Check sheet for the drawn part. Datum: minimum x, y, z corner. Units: mm. Round coordinates to 2 decimals unless told otherwise and drop trailing zeros. Write each loop counter-clockwise with the first axis right and the second up, starting at its lowest first coordinate (ties: lowest second). Pieces come first, ordered by that corner, then holes. Notation, with made-up numbers: (-34.5, -25) -> (-3.5, -25) arc R18 cw to (-3.5, -12) -> close; hole circle Ø7 at (44, 45). An arc over 180 degrees is marked (long way). One line per item, written item: value. Start each with the question number.
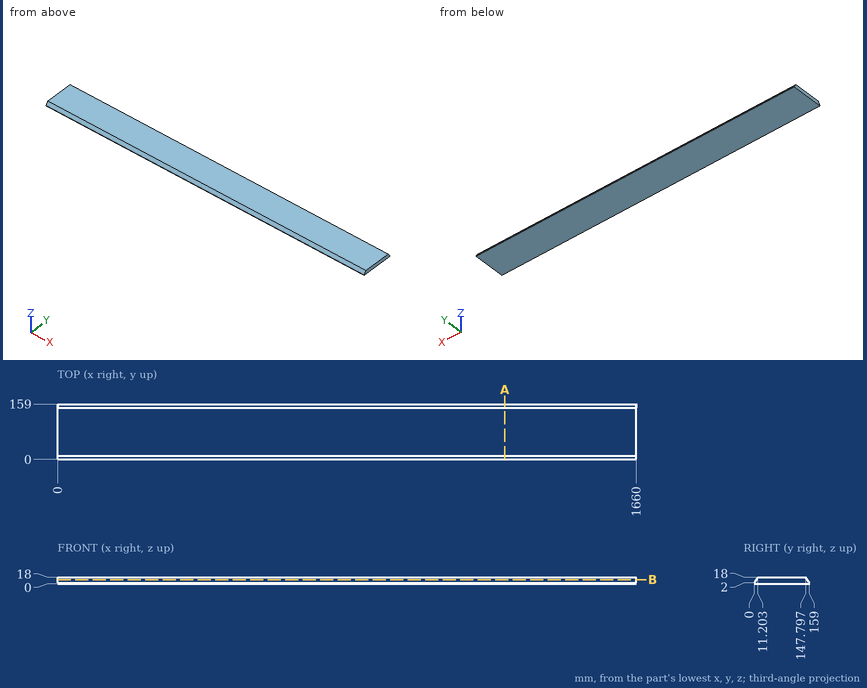
1. Cross-section at B-B (z = 11.5). Record the cut outline in (x, y), plus the area to 3 significant figures.
2. Cross-section at A-A (x = 1283.5). Record the cut outline in (y, z).
3. Material ranges on probe 1 along Y at (x, z) = (1049, 6.5); probe 2 along Y at (x, z) = (1487.5, 5), recorded low to high.
4. Depth check by flat-ended pin: pin 1 Ø3 at (x, z) = (380.5, 9) entering from +Y. Enter the tip coordinate at first touch or a pass-through.
Working result:
1. outline: (0, 6.65) -> (1660, 6.65) -> (1660, 152.35) -> (0, 152.35) -> close
1. area: 242,000 mm^2
2. outline: (0, 0) -> (159, 0) -> (159, 2) -> (147.8, 18) -> (11.2, 18) -> (0, 2) -> close
3. probe 1: y = 3.15 to 155.85
3. probe 2: y = 2.1 to 156.9
4. pin 1: stops at y = 155.15
